Geometry check sheet. Reference: drawing and pictorial views, mm from the part's lowest x, y, z. A direction names the side the tool comes from. Coordinates: 2 decimals unless noted, no trailing zeros. Write each loop counter-clockwise with the first axis right and the second up, starting at its lowest first coordinate (ties: lowest second). Pieces come first, ordered by that corner, then holes.
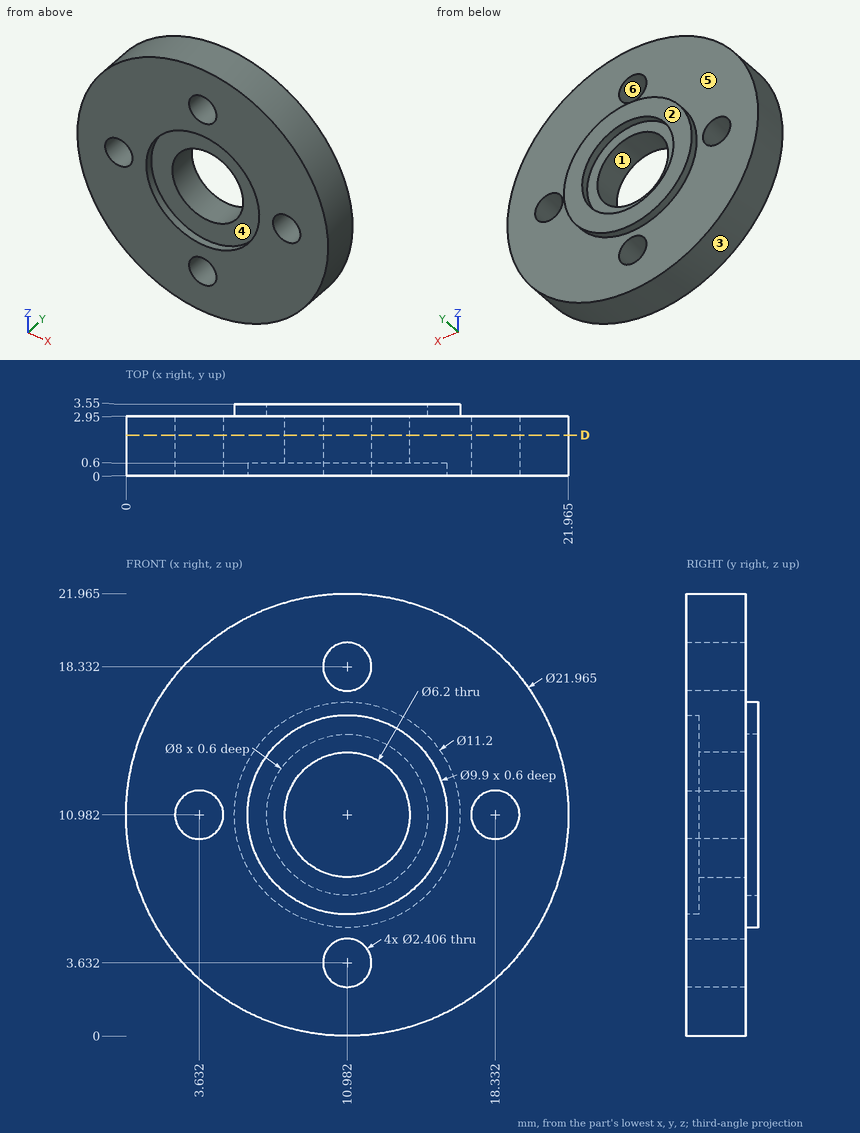
1. Sectioned sample at D-D, the plane y = 2. Record the boundary of the cut face in (x, z) (1 decimal).
2. Material ranges on L1, parallel to Y at x = 1.75, z = 10; L2, parallel to X at y = 2.25, z = 13 (1 decimal), recorded low to high.
3. Draft check along X on the marked faces 1, 2 and 3. Enter one of: pulls with the +X half, pulls with the -X half, needs draft (parallel to the pull), parting line crosses it, or undercut.
4. Tool access check on the marked faces 4, 5 and 6. Record the directions out of +Z, -Z, +X, -X, +Y, -Y that give a thin tool (end or side, any length) a straight path to the whole face; none if there is none.
5. Gauge pin test, flat ends, axial feed: P1, Ø6.5, axis at x = 10.98, z = 10.98, coming from the +Y side; P2, Ø7, axis at x = 10.98, z = 10.98, coming from the -Y side; P3, Ø3, axis at x = 18, z = 19.5, coming from the +Y side. Record the tip position at first contact, or that the pin passes through.
Outcome:
1. outline: circle Ø22 at (11, 11); hole circle Ø2.4 at (3.6, 11); hole circle Ø6.2 at (11, 11); hole circle Ø2.4 at (11, 3.6); hole circle Ø2.4 at (11, 18.3); hole circle Ø2.4 at (18.3, 11)
2. L1: y = 0 to 2.95
2. L2: x = 0.2 to 8.6, 13.3 to 21.8
3. face 1: undercut
3. face 2: needs draft
3. face 3: parting line crosses it
4. face 4: -Y
4. face 5: +Y
4. face 6: +Y, -Y
5. P1: stops at y = 2.95
5. P2: stops at y = 0.6
5. P3: stops at y = 2.95
